Read the model definition and answer for the solid it produces. Units are mm, in the model's axes. Face numbers are marked on the shaded views. A direction names the side the tool comes from. Give positions to 0.01 mm unless a question says otherwise; leave off trailing zeros. Write each loop counter-clockwise with the first axis right and the second up, starting at its lowest first coordinate (ties: lowest second). Pieces come first, ordered by that corner, then holes. Notation, with made-up numbers: (49, 51) - (76, 51) arc R20 cw to (76, 87) - close; hole circle Ø3 at (25.25, 72). An arc over 180 degrees is marked (long way). Answer as CSV lines item,"result".
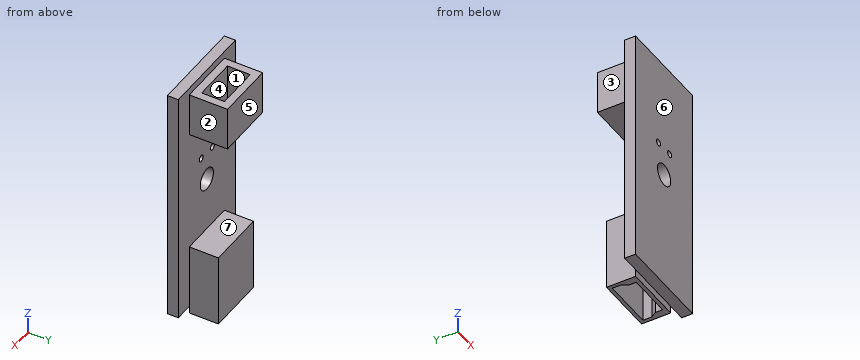
```python
from build123d import *

# Parameters (mm, degrees)
SKETCH2_W           = 13
SKETCH2_H           = 33
BOSS_EXTRUDE1_DEPTH = 1.5
SKETCH3_W           = 8
SKETCH3_H           = 6
BOSS_EXTRUDE2_DEPTH = 5.25
SKETCH4_W           = 5.878679656
SKETCH4_H           = 3.128679656
CUT_EXTRUDE1_DEPTH  = 5
SKETCH5_R           = 1.5
CUT_EXTRUDE2_DEPTH  = 7
SKETCH6_R           = 0.45
CUT_EXTRUDE3_DEPTH  = 7
SKETCH7_W           = 8
SKETCH7_H           = 9
BOSS_EXTRUDE3_DEPTH = 4
SKETCH10_W          = 8
SKETCH10_H          = 4
BOSS_EXTRUDE5_DEPTH = 1
CUT_EXTRUDE5_DEPTH  = 5


with BuildPart() as part:
    # Sketch2 → Boss-Extrude1 (new body)
    with BuildSketch(Plane(origin=(0, 0, 0), x_dir=(1, 0, 0), z_dir=(0, 1, 0))):
        Rectangle(SKETCH2_W, SKETCH2_H)
    extrude(amount=BOSS_EXTRUDE1_DEPTH)

    # Sketch3 → Boss-Extrude2 (add)
    with BuildSketch(Plane(origin=(0, 1.5, 0), x_dir=(1, 0, 0), z_dir=(0, 1, 0))):
        with Locations((0, -12.5)):
            Rectangle(SKETCH3_W, SKETCH3_H)
    extrude(amount=BOSS_EXTRUDE2_DEPTH)

    # Sketch4 → Cut-Extrude1 (cut)
    with BuildSketch(Plane.XY.offset(15.5)):
        with Locations((0, 4.125)):
            Rectangle(SKETCH4_W, SKETCH4_H)
    extrude(amount=-CUT_EXTRUDE1_DEPTH, mode=Mode.SUBTRACT)

    # Sketch5 → Cut-Extrude2 (cut)
    with BuildSketch(Plane(origin=(0, 1.5, 0), x_dir=(1, 0, 0), z_dir=(0, 1, 0))):
        with Locations(Location((0, 0, 0), (0, 0, 270))):
            Circle(SKETCH5_R)
    extrude(amount=-CUT_EXTRUDE2_DEPTH, mode=Mode.SUBTRACT)

    # Sketch6 → Cut-Extrude3 (cut)
    with BuildSketch(Plane(origin=(0, 1.5, 0), x_dir=(1, 0, 0), z_dir=(0, 1, 0))):
        with Locations(Location((-1.27, -4, 0), (0, 0, 270))):
            Circle(SKETCH6_R)
        with Locations(Location((1.27, -4, 0), (0, 0, 270))):
            Circle(SKETCH6_R)
    extrude(amount=-CUT_EXTRUDE3_DEPTH, mode=Mode.SUBTRACT)

    # Sketch7 → Boss-Extrude3 (add)
    with BuildSketch(Plane(origin=(0, 1.5, 0), x_dir=(1, 0, 0), z_dir=(0, 1, 0))):
        with Locations((0, 12)):
            Rectangle(SKETCH7_W, SKETCH7_H)
    extrude(amount=BOSS_EXTRUDE3_DEPTH)

    # Sketch10 → Boss-Extrude5 (add)
    with BuildSketch(Plane(origin=(0, 0, -16.5), x_dir=(-1, 0, 0), z_dir=(0, 0, -1))):
        with Locations((0, 3.5)):
            Rectangle(SKETCH10_W, SKETCH10_H)
    extrude(amount=BOSS_EXTRUDE5_DEPTH)

    # Sketch12 → Cut-Extrude5 (cut)
    with BuildSketch(Plane(origin=(0, 0, -17.5), x_dir=(-1, 0, 0), z_dir=(0, 0, -1))):
        Polygon((-3.490849898, 5.00909726), (3.509150102, 5.00909726), (3.509150102, 3.75909726), (3.009150102, 3.00909726), (3.009150102, 2.00909726), (-2.990849898, 2.00909726), (-2.990849898, 3.00909726), (-3.490849898, 3.75909726), align=None)
    extrude(amount=-CUT_EXTRUDE5_DEPTH, mode=Mode.SUBTRACT)


solid = part.part
```
(1) Each of these flat-tipped pins is pushed along its axis until it touches: P1, Ø1.1, axis at y = 2.5, z = -14, coming from the -X side; P2, Ø2.5, axis at x = 0.5, y = 4.5, coming from the +Z side; P3, Ø1.1, axis at y = 2.5, z = -14, coming from the +X side. Where does it stop, or does it pass through?
Worked out:
P1,"stops at x = -4"
P2,"stops at z = 15.5"
P3,"stops at x = 4"
(2) Find the intervals of material crossed by L1, parallel to X at y = 4.75, z = 12.5; L2, parallel to Z at x = 0, y = 3.5; L3, parallel to Y at x = 0.75, z = 12, in increasing order.
Worked out:
L1,"x = -4 to -2.94, 2.94 to 4"
L2,"z = -12.5 to -7.5, 9.5 to 10.5"
L3,"y = 0 to 2.56, 5.69 to 6.75"
(3) A cutting plane is placed at C-C (y = 0.5). Write down the section's boundary in (x, z).
Worked out:
outline,"(-6.5, -16.5) - (6.5, -16.5) - (6.5, 16.5) - (-6.5, 16.5) - close; hole circle Ø0.9 at (-1.27, 4); hole circle Ø3 at (0, 0); hole circle Ø0.9 at (1.27, 4)"
(4) A cutting plane is placed at B-B (z = 0). Write down the section's boundary in (x, y).
Worked out:
outline,"(-6.5, 0) - (-1.5, 0) - (-1.5, 1.5) - (-6.5, 1.5) - close; (1.5, 0) - (6.5, 0) - (6.5, 1.5) - (1.5, 1.5) - close"
(5) A cutting plane is placed at A-A (x = 0). Write down the section's boundary in (y, z), and give its area (3 significant figures).
Worked out:
outline,"(0, -16.5) - (1.5, -16.5) - (1.5, -17.5) - (2.01, -17.5) - (2.01, -12.5) - (5.01, -12.5) - (5.01, -17.5) - (5.5, -17.5) - (5.5, -7.5) - (1.5, -7.5) - (1.5, -1.5) - (0, -1.5) - close; (0, 1.5) - (1.5, 1.5) - (1.5, 9.5) - (6.75, 9.5) - (6.75, 15.5) - (5.69, 15.5) - (5.69, 10.5) - (2.56, 10.5) - (2.56, 15.5) - (1.5, 15.5) - (1.5, 16.5) - (0, 16.5) - close"
area,"85.9 mm^2"
(6) The mould has two halves that part along Y. Classify the marked faces 4, 5, 6 and 7: +Y half, -Y half, draft (parallel to the pull), parting line (faces both ways), or undercut.
Worked out:
face 4,"undercut"
face 5,"+Y half"
face 6,"-Y half"
face 7,"draft"
(7) A cutting plane is placed at D-D (z = 4). Write down the section's boundary in (x, y).
Worked out:
outline,"(-6.5, 0) - (-1.72, 0) - (-1.72, 1.5) - (-6.5, 1.5) - close; (-0.82, 0) - (0.82, 0) - (0.82, 1.5) - (-0.82, 1.5) - close; (1.72, 0) - (6.5, 0) - (6.5, 1.5) - (1.72, 1.5) - close"
(8) For the marked faces 1, 2 and 3, determine the directions among +Z, -Z, +X, -X, +Y, -Y from which every point of the face is accessible in a straight line to the end or side of a thin tool.
Worked out:
face 1,"+Z"
face 2,"+Z, -Z, +X, +Y"
face 3,"+Z, -Z, -X, +Y"
